The listing builds one solid part. Answer for the finished solid, in the listing's coordinates (mm). A direction names the side the tool comes from. Coordinates: 2 decimals unless noted, no trailing zeros. Loops run counter-clockwise (first coordinate to the right, second up) from the corner with the lowest first, then second, coordinate; pieces in that order, holes last. Notation, with made-up numbers: (-7, -1) - (46, -1) arc R23 cw to (46, 37) - close; hole circle Ø1 at (52.5, 38). An arc over 180 degrees is marked (long way). One line per question, with ' | ' between items.
from build123d import *

# Parameters (mm, degrees)
F0_W     = 950
F0_H     = 275
F1_DEPTH = 10
F2_W     = 900
F2_H     = 240
F3_DEPTH = 10
F4_W     = 200
F4_H     = 150
F5_DEPTH = 10
F6_W     = 100
F6_H     = 100
F7_DEPTH = 10


with BuildPart() as f1:
    # F0 (on Top) → F1 (new body)
    with BuildSketch(Plane.XY):
        Rectangle(F0_W, F0_H)
    extrude(amount=F1_DEPTH)

    # F2 (on face) → F3 (join)
    with BuildSketch(Plane.XZ.offset(137.5)):
        with Locations((0, -120)):
            Rectangle(F2_W, F2_H)
    extrude(amount=-F3_DEPTH)

    # F4 (on face) → F5 (cut)
    with BuildSketch(Plane.XZ.offset(137.5)):
        with Locations((-310, -165)):
            Rectangle(F4_W, F4_H)
        with Locations((0, -165)):
            Rectangle(F4_W, F4_H)
        with Locations((310, -165)):
            Rectangle(F4_W, F4_H)
    extrude(amount=-F5_DEPTH, mode=Mode.SUBTRACT)

    # F6 (on face) → F7 (cut)
    with BuildSketch(Plane.XY.offset(10)):
        with Locations((-315, 82.5)):
            Rectangle(F6_W, F6_H)
        with Locations((5, 82.5)):
            Rectangle(F6_W, F6_H)
        with Locations((325, 82.5)):
            Rectangle(F6_W, F6_H)
    extrude(amount=-F7_DEPTH, mode=Mode.SUBTRACT)


solid = f1.part
Item 1: Find section D-D, the plane x = 75.5. Write down the section's boundary in (y, z).
Taken from the geometry:
outline: (-137.5, -90) - (-127.5, -90) - (-127.5, 0) - (137.5, 0) - (137.5, 10) - (-137.5, 10) - close
Item 2: Find section A-A, the plane z = -207. Write down the section's boundary in (x, y), plus the area to 3 significant figures.
Taken from the geometry:
outline: (-450, -137.5) - (-410, -137.5) - (-410, -127.5) - (-450, -127.5) - close; (-210, -137.5) - (-100, -137.5) - (-100, -127.5) - (-210, -127.5) - close; (100, -137.5) - (210, -137.5) - (210, -127.5) - (100, -127.5) - close; (410, -137.5) - (450, -137.5) - (450, -127.5) - (410, -127.5) - close | area: 3,000 mm2
Item 3: Which of the six approach directions +Z, -Z, +X, -X, +Y, -Y give full straight-line access (tool end or side, diameter ignored) to faces 1 (the face through (-6, -127.5, -65)), 2 (the face through (-7, 2, 10))?
Taken from the geometry:
face 1: -Z, +X, -X, +Y | face 2: +Z, +X, -X, +Y, -Y
Item 4: Find section C-C, the plane y = 69.5. Write down the section's boundary in (x, z), plus the area to 3 significant figures.
Taken from the geometry:
outline: (-475, 0) - (-365, 0) - (-365, 10) - (-475, 10) - close; (-265, 0) - (-45, 0) - (-45, 10) - (-265, 10) - close; (55, 0) - (275, 0) - (275, 10) - (55, 10) - close; (375, 0) - (475, 0) - (475, 10) - (375, 10) - close | area: 6,500 mm2
Item 5: Find section B-B, the plane x = 366.5. Write down the section's boundary in (y, z), plus the area to 3 significant figures.
Taken from the geometry:
outline: (-137.5, -90) - (-127.5, -90) - (-127.5, 0) - (32.5, 0) - (32.5, 10) - (-137.5, 10) - close; (132.5, 0) - (137.5, 0) - (137.5, 10) - (132.5, 10) - close | area: 2,650 mm2
Item 6: Find the intervals of material crossed by line 1 (Z direction, x = -176.5, y = -81); line 2 (Y direction, x = 158.5, z = -100), in increasing order. Write a range as [from, to].
Taken from the geometry:
line 1: z = [0, 10] | line 2: y = [-137.5, -127.5]
Item 7: Each of these flat-tipped pins is pushed along its axis until it touches: pin 1 Ø11 at (x, y) = (355.5, -130) entering from -Z; pin 2 Ø6 at (x, y) = (63, -70) entering from -Z; pin 3 Ø8 at (y, z) = (-134.5, -155.5) entering from -X. Where does it stop, or does it pass through?
Taken from the geometry:
pin 1: stops at z = -90 | pin 2: stops at z = 0 | pin 3: stops at x = -450
